Read the model definition and answer for the solid it produces. Units are mm, in the model's axes. A direction names the side the tool comes from. Coordinates: 2 decimals unless noted, no trailing zeros. Write each loop counter-clockwise with the first axis right and the second up, starting at its lowest first coordinate (ties: lowest second). Pieces come first, ordered by that corner, then holes. Notation, with made-up numbers: (-16.75, 53) -> (18.25, 53) arc R27 ccw to (18.25, 76) -> close; hole circle Ø3 at (53.5, 56.5). An arc over 180 degrees is marked (long way). Return JSON: item names as keys, results as strings.
from build123d import *

# Parameters (mm, degrees)
SKETCH1_W             = 200
SKETCH1_H             = 300
BOSS_EXTRUDE1_DEPTH   = 12
CUT_EXTRUDE1_REACH    = 318.455
SKETCH2_W             = 90
SKETCH2_H             = 105
CUT_EXTRUDE2_REACH    = 318.455
SKETCH3_R             = 55
CUT_EXTRUDE3_REACH    = 318.455
M6X1_0_TAPPED_HOLE1_D = 5
FILLET1_R             = 20
CHAMFER1_SIZE         = 5


with BuildPart() as part:
    # Sketch1 → Boss-Extrude1 (new body)
    with BuildSketch(Plane(origin=(0, 0, 0), x_dir=(1, 0, 0), z_dir=(0, 1, 0))):
        with Locations((0, -150)):
            Rectangle(SKETCH1_W, SKETCH1_H)
    extrude(amount=BOSS_EXTRUDE1_DEPTH)

    # Sketch2 → Cut-Extrude1 (cut, up to next)
    with BuildSketch(Plane(origin=(0, 12, 0), x_dir=(1, 0, 0), z_dir=(0, 1, 0)), mode=Mode.PRIVATE) as cut_extrude1_sk1:
        with Locations((0, -247.5)):
            Rectangle(SKETCH2_W, SKETCH2_H)
    cut_extrude1_tool1 = extrude(cut_extrude1_sk1.sketch, amount=-CUT_EXTRUDE1_REACH, mode=Mode.PRIVATE) & part.part
    add(cut_extrude1_tool1.solids().sort_by_distance((0, 12, 247.5))[0], mode=Mode.SUBTRACT)

    # Sketch3 → Cut-Extrude2 (cut, up to next)
    with BuildSketch(Plane(origin=(0, 12, 0), x_dir=(1, 0, 0), z_dir=(0, 1, 0)), mode=Mode.PRIVATE) as cut_extrude2_sk1:
        with Locations(Location((0, -65, 0), (0, 0, 270))):
            Circle(SKETCH3_R)
    cut_extrude2_tool1 = extrude(cut_extrude2_sk1.sketch, amount=-CUT_EXTRUDE2_REACH, mode=Mode.PRIVATE) & part.part
    add(cut_extrude2_tool1.solids().sort_by_distance((0, 12, 65))[0], mode=Mode.SUBTRACT)

    # Sketch4 → Cut-Extrude3 (cut, up to next)
    with BuildSketch(Plane(origin=(0, 12, 0), x_dir=(1, 0, 0), z_dir=(0, 1, 0)), mode=Mode.PRIVATE) as cut_extrude3_sk1:
        with BuildLine():
            Line((-82, -268.5), (-82, -285.5))
            ThreePointArc((-82, -285.5), (-88, -291.5), (-94, -285.5))
            Line((-94, -285.5), (-94, -268.5))
            ThreePointArc((-94, -268.5), (-88, -262.5), (-82, -268.5))
        make_face()
    cut_extrude3_tool1 = extrude(cut_extrude3_sk1.sketch, amount=-CUT_EXTRUDE3_REACH, mode=Mode.PRIVATE) & part.part
    # Sketch4 → Cut-Extrude3 (cut, up to next)
    with BuildSketch(Plane(origin=(0, 12, 0), x_dir=(1, 0, 0), z_dir=(0, 1, 0)), mode=Mode.PRIVATE) as cut_extrude3_sk2:
        with BuildLine():
            Line((94, -268.5), (94, -285.5))
            ThreePointArc((94, -285.5), (88, -291.5), (82, -285.5))
            Line((82, -285.5), (82, -268.5))
            ThreePointArc((82, -268.5), (88, -262.5), (94, -268.5))
        make_face()
    cut_extrude3_tool2 = extrude(cut_extrude3_sk2.sketch, amount=-CUT_EXTRUDE3_REACH, mode=Mode.PRIVATE) & part.part
    # Sketch4 → Cut-Extrude3 (cut, up to next)
    with BuildSketch(Plane(origin=(0, 12, 0), x_dir=(1, 0, 0), z_dir=(0, 1, 0)), mode=Mode.PRIVATE) as cut_extrude3_sk3:
        with BuildLine():
            Line((-94, -176.5), (-94, -159.5))
            ThreePointArc((-94, -159.5), (-88, -153.5), (-82, -159.5))
            Line((-82, -159.5), (-82, -176.5))
            ThreePointArc((-82, -176.5), (-88, -182.5), (-94, -176.5))
        make_face()
    cut_extrude3_tool3 = extrude(cut_extrude3_sk3.sketch, amount=-CUT_EXTRUDE3_REACH, mode=Mode.PRIVATE) & part.part
    # Sketch4 → Cut-Extrude3 (cut, up to next)
    with BuildSketch(Plane(origin=(0, 12, 0), x_dir=(1, 0, 0), z_dir=(0, 1, 0)), mode=Mode.PRIVATE) as cut_extrude3_sk4:
        with BuildLine():
            Line((82, -176.5), (82, -159.5))
            ThreePointArc((82, -159.5), (88, -153.5), (94, -159.5))
            Line((94, -159.5), (94, -176.5))
            ThreePointArc((94, -176.5), (88, -182.5), (82, -176.5))
        make_face()
    cut_extrude3_tool4 = extrude(cut_extrude3_sk4.sketch, amount=-CUT_EXTRUDE3_REACH, mode=Mode.PRIVATE) & part.part
    add(cut_extrude3_tool1.solids().sort_by_distance((-88, 12, 277))[0], mode=Mode.SUBTRACT)
    add(cut_extrude3_tool2.solids().sort_by_distance((88, 12, 277))[0], mode=Mode.SUBTRACT)
    add(cut_extrude3_tool3.solids().sort_by_distance((-88, 12, 168))[0], mode=Mode.SUBTRACT)
    add(cut_extrude3_tool4.solids().sort_by_distance((88, 12, 168))[0], mode=Mode.SUBTRACT)

    # M6x1.0 Tapped Hole1 (through all)
    with Locations(Plane(origin=(0, 12, 0), x_dir=(-1, 0, 0), z_dir=(0, 1, 0))):
        with Locations((-51.265241636, 116.265241636), (51.265241636, 116.265241636), (-51.265241636, 13.734758364), (51.265241636, 13.734758364)):
            Hole(M6X1_0_TAPPED_HOLE1_D / 2)

    # Fillet1
    fillet1_edges = [part.edges().sort_by_distance(p)[0] for p in [
        (-45, 6, 195),
        (45, 6, 195),
    ]]
    fillet(fillet1_edges, radius=FILLET1_R)

    # Chamfer1
    chamfer1_edges = [part.edges().sort_by_distance(p)[0] for p in [
        (-45, 6, 300),
        (45, 6, 300),
        (-100, 6, 0),
        (100, 6, 0),
        (100, 6, 300),
        (-100, 6, 300),
    ]]
    chamfer(chamfer1_edges, length=CHAMFER1_SIZE)


solid = part.part
1. The part is cut by section D-D (y = 2.5). Count the separate pieces of the cut face and the enclosed holes in it, then the cut area to 3 significant figures.
Taken from the geometry:
{"separate pieces": "1", "enclosed holes": "9", "area": "39,800 mm2"}
2. The part is cut by section B-B (z = 65). Determine the outline of the cut face in (x, y).
Taken from the geometry:
{"outline": "(-100, 0) -> (-55, 0) -> (-55, 12) -> (-100, 12) -> close; (55, 0) -> (100, 0) -> (100, 12) -> (55, 12) -> close"}
3. Consider L1, parallel to X at y = 4, z = 249.5; L2, parallel to X at y = 4.25, z = 283.5; L3, parallel to Z at x = -84.5, y = 2. Determine where each line is inside the solid, lowest interval first.
Taken from the geometry:
{"L1": "x = -100 to -45, 45 to 100", "L2": "x = -100 to -94, -82 to -45, 45 to 82, 94 to 100", "L3": "z = 0 to 154.63, 181.37 to 263.63, 290.37 to 300"}
4. For a pull along X with two mould halves and no side action, classify faces 1 (the face through (-39.297, 5.916, 201.014)), 2 (the face through (-1, 12, 148)), 3 (the face through (100, 6, 152)) as +X half, -X half, draft (parallel to the pull), parting line (faces both ways), or undercut.
Taken from the geometry:
{"face 1": "undercut", "face 2": "draft", "face 3": "+X half"}
5. The part is cut by section A-A (x = -88). Determine the outline of the cut face in (y, z), then the cut area to 3 significant figures.
Taken from the geometry:
{"outline": "(0, 0) -> (12, 0) -> (12, 153.5) -> (0, 153.5) -> close; (0, 182.5) -> (12, 182.5) -> (12, 262.5) -> (0, 262.5) -> close; (0, 291.5) -> (12, 291.5) -> (12, 300) -> (0, 300) -> close", "area": "2,900 mm2"}
6. A flat-ended cylindrical pin translates along its axis: pin 1 Ø8 at (x, z) = (51.27, 13.73) entering from +Y. Find the tip coordinate at first contact, or state that the pin passes through.
Taken from the geometry:
{"pin 1": "stops at y = 12"}
7. A tool of negligible diameter and unlimited length cuts with its end or side. For faces 4 (the face through (-100, 6, 152)), 5 (the face through (82, 6, 277)), 6 (the face through (38.986, 5.916, 200.703)), from which of +Z, -Z, +X, -X, +Y, -Y can it reach the whole face along a straight path? Write none if from no direction.
Taken from the geometry:
{"face 4": "+Z, -Z, -X, +Y, -Y", "face 5": "+Y, -Y", "face 6": "+Z, +Y, -Y"}
8. The part is cut by section C-C (x = 0). Determine the outline of the cut face in (y, z).
Taken from the geometry:
{"outline": "(0, 0) -> (12, 0) -> (12, 10) -> (0, 10) -> close; (0, 120) -> (12, 120) -> (12, 195) -> (0, 195) -> close"}
